from build123d import *

# Parameters (mm, degrees)
SKETCH1_W           = 10.16
SKETCH1_H           = 7.239
BOSS_EXTRUDE1_DEPTH = 7.112
FILLET2_R           = 0.254
FILLET3_R           = 0.127


with BuildPart() as part:
    # Sketch1 → Boss-Extrude1 (new body, symmetric)
    with BuildSketch(Plane.XY):
        Polygon((0, 8.6995), (5.08, 3.6195), (-5.08, 3.6195), align=None)
        Rectangle(SKETCH1_W, SKETCH1_H)
    extrude(amount=BOSS_EXTRUDE1_DEPTH, both=True)

    # Fillet2
    fillet2_edges = [part.edges().sort_by_distance(p)[0] for p in [
        (5.08, 3.6195, 0),
        (-5.08, 3.6195, 0),
    ]]
    fillet(fillet2_edges, radius=FILLET2_R)

    # Fillet3
    fillet3_edges = [part.edges().sort_by_distance(p)[0] for p in [
        (0, 8.6995, 0),
    ]]
    fillet(fillet3_edges, radius=FILLET3_R)


solid = part.part
Geometry check sheet. Reference: the model listing, model coordinates, mm. Round coordinates to 2 decimals unless told otherwise and drop trailing zeros. Order: outer loops, then holes, each group sorted by start corner. A loop starts at its lowest first (then second) coordinate and runs counter-clockwise, first axis right, second up. Notation, with made-up numbers: M -30.5,55.25 L 23.5,55.25 A11 cw 23.5,60.25 Z; hole C -37,-25 d3. An arc over 180 degrees is marked long. Answer in a Markdown table with one row per item.
(1) Sectioned sample at A-A, the plane z = -6. Record the cut outline in (x, y), and give its area (3 significant figures).
Responses:
| item | result |
|---|---|
| outline | M -5.08,-3.62 L 5.08,-3.62 L 5.08,3.51 A0.25 ccw 5.01,3.69 L 0.09,8.61 A0.13 ccw -0.09,8.61 L -5.01,3.69 A0.25 ccw -5.08,3.51 Z |
| area | 99.3 mm² |
(2) Sectioned sample at C-C, the plane y = 5.5. Record the cut outline in (x, z).
Responses:
| item | result |
|---|---|
| outline | M -3.2,-7.11 L 3.2,-7.11 L 3.2,7.11 L -3.2,7.11 Z |
(3) Sectioned sample at B-B, the plane x = 3.75. Record the cut outline in (y, z).
Responses:
| item | result |
|---|---|
| outline | M -3.62,-7.11 L 4.95,-7.11 L 4.95,7.11 L -3.62,7.11 Z |
(4) Scan lines: probe 1 along X at (y, z) = (8, 5.25); probe 2 along Y at (x, z) = (4, -6.5); probe 3 along Y at (x, z) = (2, -1.25). Record each from-to range of solid material in increasing order. Write a range as from..to.
Responses:
| item | result |
|---|---|
| probe 1 | x = -0.7..0.7 |
| probe 2 | y = -3.62..4.7 |
| probe 3 | y = -3.62..6.7 |
(5) Go/stop test with a flat-tipped pin: P1, Ø1.5, axis at x = -3.5, z = 1.5, coming from the +Y side. Record where the tip stops, or that it passes through.
Responses:
| item | result |
|---|---|
| P1 | stops at y = 5.95 |
